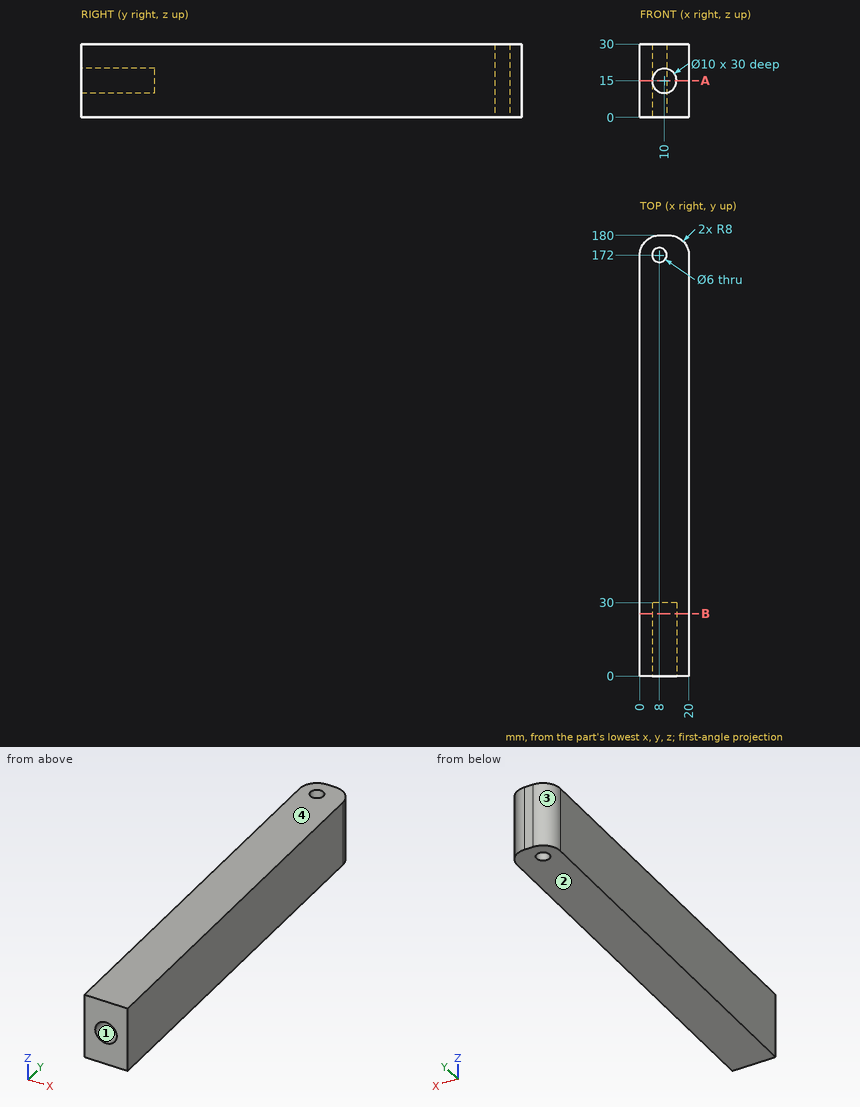
Study the drawing (mm; zero at the part's minimum x, y, z) and answer. Round coordinates to 2 decimals unless told otherwise and drop trailing zeros. Write each loop counter-clockwise with the first axis right and the second up, starting at its lowest first coordinate (ties: lowest second). Pieces come first, ordered by that corner, then holes. Notation, with made-up numbers: (65.25, 21.25) - (86.25, 21.25) arc R33 cw to (86.25, 54.25) - close; hole circle Ø5 at (-12.5, 48). An arc over 180 degrees is marked (long way). Use a Markdown table: item, result. Add a question column.
1. Consider line 1 (X direction, y = 19.75, z = 15); line 2 (Y direction, x = 8, z = 9.25); line 3 (Y direction, x = 8, z = 14.5). Determine where each line is inside the solid, lowest interval first.
2. The part is cut by section A-A (z = 15). Write down the section's boundary in (x, y), and give its area (3 significant figures).
3. Flat-ended cylindrical pins translate along their axes: P1, Ø3, axis at x = 11, z = 14.5, coming from the -Y side; P2, Ø1.5, axis at x = 13, z = 12.5, coming from the +Y side; P3, Ø5, axis at x = 16.5, z = 22, coming from the +Y side. Find the tip coordinate at first contact, or state that the pin passes through.
4. The part is cut by section B-B (y = 25.5). Write down the section's boundary in (x, z).
5. For a pull along Z with two mould halves and no side action, classify the marked faces 1, 2, 3 and 4 as +Z half, -Z half, draft (parallel to the pull), parting line (faces both ways), or undercut.
Reported:
| question | item | result |
|---|---|---|
| 1 | line 1 | 0 to 5, 15 to 20 |
| 1 | line 2 | 0 to 169, 175 to 180 |
| 1 | line 3 | 30 to 169, 175 to 180 |
| 2 | outline | (0, 0) - (5, 0) - (5, 30) - (15, 30) - (15, 0) - (20, 0) - (20, 172) arc R8 ccw to (12, 180) - (8, 180) arc R8 ccw to (0, 172) - close; hole circle Ø6 at (8, 172) |
| 2 | area | 3,240 mm^2 |
| 3 | P1 | y = 30 |
| 3 | P2 | y = 180 |
| 3 | P3 | y = 179.75 |
| 4 | outline | (0, 0) - (20, 0) - (20, 30) - (0, 30) - close; hole circle Ø10 at (10, 15) |
| 5 | face 1 | undercut |
| 5 | face 2 | -Z half |
| 5 | face 3 | draft |
| 5 | face 4 | +Z half |
